Design review of the part built by this model. Coordinates are the model's own, in mm. Face numbers are marked on the shaded views. A direction names the side the tool comes from. Give positions to 0.01 mm unless a question says otherwise; leave off trailing zeros. Write each loop counter-clockwise with the first axis right and the second up, starting at its lowest first coordinate (ties: lowest second). Pieces come first, ordered by that corner, then holes. Notation, with made-up numbers: M 0,78 L 26,78 A15 cw 26,107 Z; hole C 58.25,87 d3. An arc over 180 degrees is marked long. One line per item, written item: value. Start each with the question number.
```python
from build123d import *

# Parameters (mm, degrees)
EXTRUDE_1_DEPTH          = 9.5
CUT_EXTRUDE_1_DEPTH      = 2
CUT_EXTRUDE_2_DEPTH      = 5
CUT_EXTRUDE_2_DEPTH_BACK = 5
CHAMFER_3_SIZE           = 0.2
CHAMFER_4_SIZE           = 0.2
CHAMFER_5_SIZE           = 0.2
SKETCH_35_R              = 1.52
CUT_EXTRUDE_3_DEPTH      = 2


with BuildPart() as part:
    # Sketch 1 → Extrude 1 (new body)
    with BuildSketch(Plane.XY.offset(14.66)):
        with BuildLine():
            Line((10.013875018, 11.640660484), (26.695757592, 11.640660484))
            ThreePointArc((26.695757592, 11.640660484), (29.763542255, 12.692408053), (31.540712894, 15.405181579))
            ThreePointArc((31.540712894, 15.405181579), (31.567392591, 15.532704372), (31.582905999, 15.662061255))
            ThreePointArc((31.582905999, 15.662061255), (30.767257841, 17.705140503), (28.652721603, 18.311928133))
            ThreePointArc((28.652721603, 18.311928133), (28.148188919, 18.150812525), (27.70363757, 17.86291399))
            ThreePointArc((27.70363757, 17.86291399), (26.793087906, 17.328646623), (25.753839798, 17.142889571))
            Line((25.753839798, 17.142889571), (22.790573212, 17.142889571))
            ThreePointArc((22.790573212, 17.142889571), (20.202578582, 17.48357884), (17.790924351, 18.482432813))
            Line((17.790924351, 18.482432813), (17.43600444, 18.687326732))
            ThreePointArc((17.43600444, 18.687326732), (16.230177325, 19.186753718), (14.93618001, 19.357098353))
            Line((14.93618001, 19.357098353), (9.471737064, 19.357098353))
            ThreePointArc((9.471737064, 19.357098353), (6.685692146, 19.552100152), (3.953975606, 20.133302981))
            Line((3.953975606, 20.133302981), (3.531774948, 20.254486258))
            ThreePointArc((3.531774948, 20.254486258), (0.800058407, 20.835689087), (-1.985986511, 21.030690887))
            Line((-1.985986511, 21.030690887), (-15.538147248, 21.030690887))
            ThreePointArc((-15.538147248, 21.030690887), (-20.108103219, 18.591001725), (-20.623778443, 13.436328132))
            ThreePointArc((-20.623778443, 13.436328132), (-19.195597321, 7.592016854), (-19.570086215, 1.587399156))
            ThreePointArc((-19.570086215, 1.587399156), (-18.531135486, -4.083088818), (-13.775230647, -7.341189744))
            Line((-13.775230647, -7.341189744), (-11.288176227, -6.122720263))
            Line((-11.288176227, -6.122720263), (-10.853623376, -4.518995222))
            ThreePointArc((-10.853623376, -4.518995222), (-7.637616135, -1.077692314), (-8.991428746, 3.433677732))
            Line((-8.991428746, 3.433677732), (-5.185613362, 5.521767908))
            ThreePointArc((-5.185613362, 5.521767908), (-4.30923615, 6.249201579), (-3.767164175, 7.250877543))
            Line((-3.767164175, 7.250877543), (-3.486450124, 8.142372809))
            ThreePointArc((-3.486450124, 8.142372809), (-1.67460917, 10.672320293), (1.282707044, 11.640660484))
            Line((1.282707044, 11.640660484), (10.013875018, 11.640660484))
        make_face()
    extrude(amount=-EXTRUDE_1_DEPTH)

    # Sketch 2 → Cut-Extrude 1 (cut)
    with BuildSketch(Plane.XY.offset(14.66)):
        with BuildLine():
            ThreePointArc((-18.576270357, 1.449716513), (-10.888967052, -6.358042936), (-7.040699486, 3.900932474))
            ThreePointArc((-7.040699486, 3.900932474), (-9.967136502, 9.432986631), (-11.040523791, 15.598657441))
            ThreePointArc((-11.040523791, 15.598657441), (-14.604669497, 11.128277968), (-19.678620032, 13.763131518))
            ThreePointArc((-19.678620032, 13.763131518), (-18.152154257, 7.693736239), (-18.576270357, 1.449716513))
        make_face()
    extrude(amount=-CUT_EXTRUDE_1_DEPTH, mode=Mode.SUBTRACT)

    # Sketch 7 → Cut-Extrude 2 (cut, two sides)
    with BuildSketch(Plane.XY.offset(12.16)) as cut_extrude_2_sk:
        with BuildLine():
            Line((-11.093260582, -6.093027877), (-10.743074352, -4.770661757))
            ThreePointArc((-10.743074352, -4.770661757), (-7.437188108, -1.39032296), (-8.426086578, 3.233274564))
            ThreePointArc((-8.426086578, 3.233274564), (-7.84768541, 3.478159198), (-7.255220155, 3.686728888))
            ThreePointArc((-7.255220155, 3.686728888), (-18.011463654, 2.26499609), (-11.093260582, -6.093027877))
        make_face()
    extrude(amount=CUT_EXTRUDE_2_DEPTH, mode=Mode.SUBTRACT)
    extrude(cut_extrude_2_sk.sketch, amount=-CUT_EXTRUDE_2_DEPTH_BACK, mode=Mode.SUBTRACT)

    # Sketch 20 → Cut-Revolve 1 (revolve, cut)
    with BuildSketch(Plane(origin=(0, 15.5, 0), x_dir=(1, 0, 0), z_dir=(0, 1, 0))):
        Polygon((-13.84, -5.16), (-15.54, -5.16), (-15.54, -14.66), (-11.04, -14.66), (-11.04, -9.16), (-13.84, -9.16), align=None)
    revolve(axis=Axis((-15.54, 15.5, 5.16), (0, 0, 1)), mode=Mode.SUBTRACT)

    # Sketch 28 → Revolve 1 (revolve)
    with BuildSketch(Plane(origin=(0, 0, 9.91), x_dir=(-1, 0, 0), z_dir=(0, 0, -1))):
        with BuildLine():
            Line((-15.045898034, 9.140660484), (-14.15, 9.140660484))
            Line((-14.15, 9.140660484), (-14.15, 11.640660484))
            Line((-14.15, 11.640660484), (-18.65, 11.640660484))
            Line((-18.65, 11.640660484), (-18.021509962, 11.424042656))
            ThreePointArc((-18.021509962, 11.424042656), (-17.642565022, 11.188030722), (-17.404086822, 10.81063299))
            ThreePointArc((-17.404086822, 10.81063299), (-16.490704468, 9.600431485), (-15.045898034, 9.140660484))
        make_face()
    revolve(axis=Axis((14.15, 9.140660484, 9.91), (0, 1, 0)))

    # Sketch 31 → Revolve 2 (revolve)
    with BuildSketch(Plane(origin=(0, 0, 0), x_dir=(1, 0, 0), z_dir=(0, 1, 0))):
        Polygon((-8.477724428, -7.16), (-12.24, -7.16), (-12.24, -7.751660878), (-10.2, -7.751660878), (-8.916332066, -7.751660878), align=None)
    revolve(axis=Axis((-12.24, 0, 7.16), (0, 0, 1)))

    # Sketch 34 → Cut-Revolve 2 (revolve, cut)
    with BuildSketch(Plane(origin=(-5.952118717, 0.015774741, 0), x_dir=(0, 0, -1), z_dir=(0.99998395, 0.005665598, 0))):
        Polygon((-9.91, 21.068889451), (-9.91, 4.068889451), (-8.61, 4.068889451), (-8.11, 16.068889451), (-5.91, 21.068889451), align=None)
    revolve(axis=Axis((-6.575334536, 110.014009282, 9.91), (0.005665598, -0.99998395, 0)), mode=Mode.SUBTRACT)

    # Chamfer 3
    chamfer_3_edges = [part.edges().sort_by_distance(p)[0] for p in [
        (-4.30923615, 6.249201579, 5.16),
        (-3.626807149, 7.696625176, 5.16),
        (-1.67460917, 10.672320293, 5.16),
        (13.989232318, 11.640660484, 5.16),
        (29.763542255, 12.692408053, 5.16),
        (31.567392591, 15.532704372, 5.16),
        (30.767257841, 17.705140503, 5.16),
        (28.148188919, 18.150812525, 5.16),
        (26.793087906, 17.328646623, 5.16),
        (-7.637616135, -1.077692314, 5.16),
        (24.272206505, 17.142889571, 5.16),
        (20.202578582, 17.48357884, 5.16),
        (17.613464396, 18.584879772, 5.16),
        (16.230177325, 19.186753718, 5.16),
        (12.203958537, 19.357098353, 5.16),
        (6.685692146, 19.552100152, 5.16),
        (3.742875277, 20.19389462, 5.16),
        (0.800058407, 20.835689087, 5.16),
        (-8.762066879, 21.030690887, 5.16),
        (-20.108103219, 18.591001725, 5.16),
        (-7.088521054, 4.47772282, 5.16),
        (-19.195597321, 7.592016854, 5.16),
        (-18.531135486, -4.083088818, 5.16),
        (-12.531703437, -6.731955004, 5.16),
        (-11.070899801, -5.320857743, 5.16),
    ]]
    chamfer(chamfer_3_edges, length=CHAMFER_3_SIZE)

    # Chamfer 4
    chamfer_4_edges = [part.edges().sort_by_distance(p)[0] for p in [
        (-17.24, 15.5, 5.16),
    ]]
    chamfer(chamfer_4_edges, length=CHAMFER_4_SIZE)

    # Chamfer 5
    chamfer_5_edges = [part.edges().sort_by_distance(p)[0] for p in [
        (-18.531135486, -4.083088818, 14.66),
        (-19.195597321, 7.592016854, 14.66),
        (-20.108103219, 18.591001725, 14.66),
        (-8.762066879, 21.030690887, 14.66),
        (0.800058407, 20.835689087, 14.66),
        (3.742875277, 20.19389462, 14.66),
        (6.685692146, 19.552100152, 14.66),
        (12.203958537, 19.357098353, 14.66),
        (16.230177325, 19.186753718, 14.66),
        (17.613464396, 18.584879772, 14.66),
        (20.202578582, 17.48357884, 14.66),
        (24.272206505, 17.142889571, 14.66),
        (26.793087906, 17.328646623, 14.66),
        (28.148188919, 18.150812525, 14.66),
        (30.767257841, 17.705140503, 14.66),
        (31.567392591, 15.532704372, 14.66),
        (29.763542255, 12.692408053, 14.66),
        (13.989232318, 11.640660484, 14.66),
        (-1.67460917, 10.672320293, 14.66),
        (-3.626807149, 7.696625176, 14.66),
        (-4.30923615, 6.249201579, 14.66),
        (-6.270263103, 4.926666401, 14.66),
    ]]
    chamfer(chamfer_5_edges, length=CHAMFER_5_SIZE)

    # Sketch 35 → Cut-Extrude 3 (cut)
    with BuildSketch(Plane.XY.offset(7.751660878)):
        with Locations((-12.24, 0)):
            Circle(SKETCH_35_R)
    extrude(amount=-CUT_EXTRUDE_3_DEPTH, mode=Mode.SUBTRACT)


solid = part.part
```
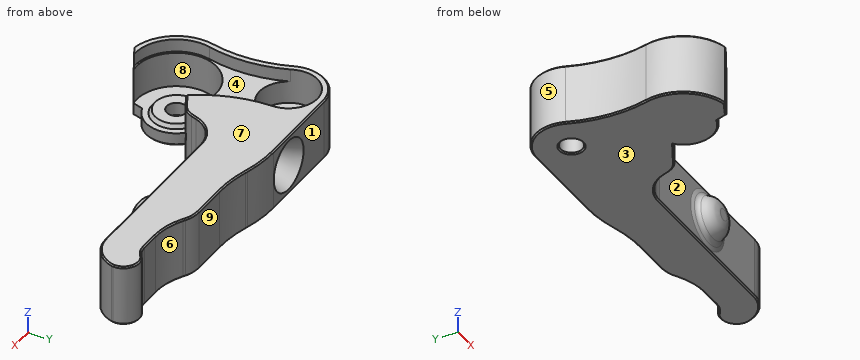
Q1. For P1, Ø1, axis at x = -7.5, z = 10, coming from the +Y side; P2, Ø3.5, axis at x = -12, y = 0.5, coming from the +Z side; P3, Ø4.5, axis at x = 11.5, z = 8, coming from the -Y side, all flat-tipped, find the tip position at first contact; note any pin that passes through.
Q2. Wall thickness on line 1 (Y direction, x = -15.54, z = 8.4); line 2 (Y direction, x = -15.54, z = 10.7); line 3 (Y direction, x = 23.5, z = 6): over which ranges is each line inside the solid? List them lowest first. Write a range as from..to.
Q3. Take a section at B-B, the plane z = 9.91. State how many separate pieces and enclosed holes the cut face has, then the cut area to 3 significant figures.
Q4. The part is to be moulded in two halves that separate along Y. For the marked faces 1, 2, 3 and 4, say which applies: pulls with the +Y half, pulls with the -Y half, needs draft (parallel to the pull), parting line crosses it, or undercut.
Q5. Take a section at A-A, the plane y = 0. Give the boundary of the cut face in (x, z), then the cut area to 3 significant figures.
Q6. Machinability: for the marked faces 5, 6, 7, 8 and 9, which of the approach directions +Z, -Z, +X, -X, +Y, -Y give a long, thin tool a straight path to every point of the face, cutting with its end or side? Answer none if there is none.
Results list:
1. P1: stops at y = 16.43
1. P2: stops at z = 7.75
1. P3: stops at y = 9.14
2. line 1: y = -6.73..-5.25, 5.25..13.8, 17.2..21.03
2. line 2: y = -6.73..-5.25, 5.25..11, 20..21.03
2. line 3: y = 11.64..17.14
3. separate pieces: 2
3. enclosed holes: 1
3. area: 421 mm^2
4. face 1: pulls with the +Y half
4. face 2: pulls with the -Y half
4. face 3: needs draft
4. face 4: undercut
5. outline: M -19.74,5.36 L -19.54,5.16 L -7.71,5.16 L -7.51,5.36 L -7.51,7.16 L -8.48,7.16 L -8.92,7.75 L -10.72,7.75 L -10.72,5.75 L -13.76,5.75 L -13.76,7.75 L -15.56,7.75 L -16,7.16 L -18.44,7.16 L -18.44,12.66 L -18.74,12.66 L -18.74,14.66 L -19.54,14.66 L -19.74,14.46 Z
5. area: 31.7 mm^2
6. face 5: +Z, -Z, -X
6. face 6: +Z, -Z, +Y
6. face 7: +Z, +X, -X, +Y, -Y
6. face 8: +Z
6. face 9: +Z, -Z, +X, +Y
